CAD build for the part. Positions are in the model's coordinates, mm. Face numbers are marked on the shaded views. A direction names the side the tool comes from. Give positions to 0.01 mm unless a question says otherwise; leave off trailing zeros. Order: outer loops, then holes, each group sorted by start corner. A loop starts at its lowest first (then second) coordinate and runs counter-clockwise, first axis right, second up. Notation, with made-up numbers: M 32.5,30 L 88.5,30 A22 cw 88.5,64 Z; hole C -38.5,76.5 d7. An arc over 180 degrees is marked long. Put each result on its own line as item: value. Start each with the question number.
1) Cut at C-C (y = -77). Write the cut outline in (x, z).
2) Cut at B-B (z = 2). Write the cut outline in (x, y).
3) Pin check, flat tips, straight feed: pin 1 (1.6 mm diameter, centred on x = 2.5, z = 2.5, fed in from -Y); pin 2 (1.6 mm diameter, centred on y = -14, z = 3, fed in from -X). Stop position of each tip, or through.
4) Drill centre lines: line 1 (Y direction, x = 5.25, z = 4.5); line 2 (X direction, y = -91.5, z = 5.1). Where is each one in solid material? Low to high. Write a range as [from, to].
5) Cut at A-A (x = 2.5). Write the cut outline in (y, z), and give its area (3 significant figures).
6) Two-plate mould, pull along Y, no slides. Class the marked faces 3, 4, 5 and 6: released by +Y, released by -Y, zero draft, split by the parting line, or undercut.
7) Tool access for the marked faces 1 and 2: list every direction of +Z, -Z, +X, -X, +Y, -Y with a clear straight run to the whole face (end or side of a thin tool).
```python
from build123d import *

# Parameters (mm, degrees)
SKETCH_1_W          = 14.5
SKETCH_1_H          = 100
EXTRUDE_1_DEPTH     = 5.5
SKETCH_2_W          = 5.5
SKETCH_2_H          = 10
CUT_EXTRUDE_1_DEPTH = 102.195355625


with BuildPart() as part:
    # ｽｹｯﾁ1 → ﾎﾞｽ - 押し出し1 (new body)
    with BuildSketch(Plane.XY):
        with Locations((7.25, -50)):
            Rectangle(SKETCH_1_W, SKETCH_1_H)
    extrude(amount=EXTRUDE_1_DEPTH)

    # ｽｹｯﾁ2 → ｶｯﾄ - 押し出し1 (cut, through all)
    with BuildSketch(Plane.XY.offset(5.5)):
        with Locations((2.75, -15)):
            Rectangle(SKETCH_2_W, SKETCH_2_H)
        with Locations((2.75, -35)):
            Rectangle(SKETCH_2_W, SKETCH_2_H)
        with Locations((2.75, -55)):
            Rectangle(SKETCH_2_W, SKETCH_2_H)
        with Locations((2.75, -75)):
            Rectangle(SKETCH_2_W, SKETCH_2_H)
        with Locations((2.75, -95)):
            Rectangle(SKETCH_2_W, SKETCH_2_H)
    extrude(amount=-CUT_EXTRUDE_1_DEPTH, mode=Mode.SUBTRACT)


solid = part.part
```
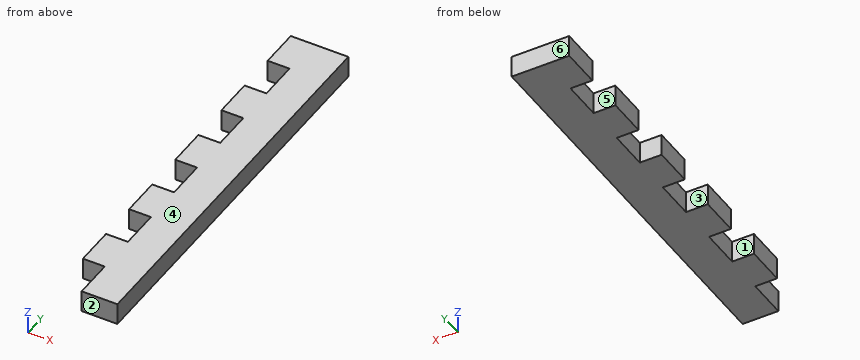
Solution:
1. outline: M 5.5,0 L 14.5,0 L 14.5,5.5 L 5.5,5.5 Z
2. outline: M 0,-90 L 5.5,-90 L 5.5,-100 L 14.5,-100 L 14.5,0 L 0,0 L 0,-10 L 5.5,-10 L 5.5,-20 L 0,-20 L 0,-30 L 5.5,-30 L 5.5,-40 L 0,-40 L 0,-50 L 5.5,-50 L 5.5,-60 L 0,-60 L 0,-70 L 5.5,-70 L 5.5,-80 L 0,-80 Z
3. pin 1: y = -90
3. pin 2: x = 5.5
4. line 1: [-90, -80], [-70, -60], [-50, -40], [-30, -20], [-10, 0]
4. line 2: [5.5, 14.5]
5. outline: M -90,0 L -80,0 L -80,5.5 L -90,5.5 Z; M -70,0 L -60,0 L -60,5.5 L -70,5.5 Z; M -50,0 L -40,0 L -40,5.5 L -50,5.5 Z; M -30,0 L -20,0 L -20,5.5 L -30,5.5 Z; M -10,0 L 0,0 L 0,5.5 L -10,5.5 Z
5. area: 275 mm²
6. face 3: undercut
6. face 4: zero draft
6. face 5: undercut
6. face 6: released by +Y
7. face 1: +Z, -Z, -X
7. face 2: +Z, -Z, +X, -X, -Y
